Verification items for the finished model (mm, model axes). Face numbers are marked on the shaded views. A direction names the side the tool comes from. Give positions to 0.01 mm unless a question says otherwise; leave off trailing zeros. Write each loop counter-clockwise with the first axis right and the second up, starting at its lowest first coordinate (ties: lowest second). Pieces come first, ordered by that corner, then holes. Notation, with made-up numbers: (77.5, -27) -> (86.5, -27) arc R12 ccw to (86.5, -5) -> close; hole circle Ø4 at (-26, 55). An arc over 180 degrees is marked (long way). Write item = value, one per line.
from build123d import *

# Parameters (mm, degrees)
BOX009_W          = 12
BOX009_H          = 12
BOX009_DEPTH      = 4
CYLINDER003_R     = 3.5
CYLINDER003_DEPTH = 5


with BuildPart() as obj1:
    # Box009 → Box009 (new body)
    with BuildSketch(Plane.XY):
        with Locations((6, 6)):
            Rectangle(BOX009_W, BOX009_H)
    extrude(amount=BOX009_DEPTH)


with BuildPart() as button:
    # Cylinder003 → Cylinder003 (new body)
    with BuildSketch(Plane(origin=(6, 6, 4), x_dir=(1, 0, 0), z_dir=(0, 0, 1))):
        Circle(CYLINDER003_R)
    extrude(amount=CYLINDER003_DEPTH)

    # Fusion001: union obj1
    add(obj1.part)


with BuildPart() as button_1:
    # Fusion001 placement: moved
    add(button.part.moved(Location((52, 92, 1.1))))


solid = button_1.part
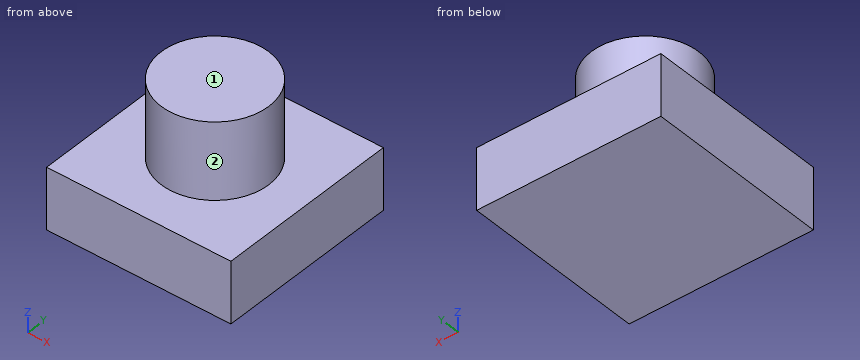
Item 1: Sectioned sample at D-D on y = 93.25. Record the cut outline in (x, z).
Response values:
outline = (52, 1.1) -> (64, 1.1) -> (64, 5.1) -> (52, 5.1) -> close
Item 2: Set-up check for the marked faces 1 and 2: record each of +Z, -Z, +X, -X, +Y, -Y from which the full face is reachable in a straight line by a thin tool's end or side.
Response values:
face_1 = +Z, +X, -X, +Y, -Y
face_2 = +Z
Item 3: Material ranges on line 1 (Z direction, x = 54, y = 93.75); line 2 (Y direction, x = 58, z = 9.75); line 3 (X direction, y = 97.5, z = 7), recorded low to high.
Response values:
line_1 = 1.1 to 5.1
line_2 = 94.5 to 101.5
line_3 = 54.54 to 61.46
Item 4: Sectioned sample at A-A on x = 58. Record the cut outline in (y, z).
Response values:
outline = (92, 1.1) -> (104, 1.1) -> (104, 5.1) -> (101.5, 5.1) -> (101.5, 10.1) -> (94.5, 10.1) -> (94.5, 5.1) -> (92, 5.1) -> close
Item 5: Sectioned sample at C-C on z = 6.75. Record the cut outline in (x, y).
Response values:
outline = circle Ø7 at (58, 98)
Item 6: Sectioned sample at B-B on y = 100.75. Record the cut outline in (x, z).
Response values:
outline = (52, 1.1) -> (64, 1.1) -> (64, 5.1) -> (60.17, 5.1) -> (60.17, 10.1) -> (55.83, 10.1) -> (55.83, 5.1) -> (52, 5.1) -> close
Item 7: Go/stop test with flat-tipped pins: P1, Ø4, axis at x = 61.5, z = 8.5, coming from the +Y side; P2, Ø4, axis at x = 54.5, z = 8, coming from the -Y side. Record where each tip stops, or that it passes through.
Response values:
P1 = 101.16
P2 = 94.84
